from build123d import *
from build123d.topology import SkipClean

# Parameters (mm, degrees)
SKETCH1_W                = 60
SKETCH1_H                = 30
SKETCH1_R                = 11.5
BOSS_EXTRUDE1_DEPTH      = 5
SKETCH2_R                = 1.6
CUT_EXTRUDE1_DEPTH       = 68.268120235
FILLET1_R                = 5
SKETCH6_R                = 1.6
SKETCH6_R_2              = 11.5
BOSS_EXTRUDE4_DEPTH      = 3
FILLET1_OF_MIRROR1_R     = 5
SKETCH7_W                = 8
SKETCH7_H                = 5
BOSS_EXTRUDE5_DEPTH      = 8
CHAMFER1_SIZE            = 7
CHAMFER1_OF_MIRROR2_SIZE = 7


with BuildPart() as part:
    # Sketch1 → Boss-Extrude1 (new body)
    with BuildSketch(Plane(origin=(0, 0, 0), x_dir=(1, 0, 0), z_dir=(0, 1, 0))):
        with Locations((30, 15)):
            Rectangle(SKETCH1_W, SKETCH1_H)
        with Locations(Location((22, 15, 0), (0, 0, 270))):
            Circle(SKETCH1_R, mode=Mode.SUBTRACT)
    boss_extrude1 = extrude(amount=BOSS_EXTRUDE1_DEPTH)

    # Sketch2 → Cut-Extrude1 (cut, through all)
    with BuildSketch(Plane(origin=(0, 5, 0), x_dir=(1, 0, 0), z_dir=(0, 1, 0))):
        with Locations(Location((56, 25, 0), (0, 0, 270))):
            Circle(SKETCH2_R)
        with Locations(Location((56, 5, 0), (0, 0, 270))):
            Circle(SKETCH2_R)
    cut_extrude1 = extrude(amount=-CUT_EXTRUDE1_DEPTH, mode=Mode.SUBTRACT)

    # Fillet1
    fillet1_edges = [part.edges().sort_by_distance(p)[0] for p in [
        (0, 2.5, -30),
        (0, 2.5, 0),
    ]]
    fillet(fillet1_edges, radius=FILLET1_R)

    # Sketch6 → Boss-Extrude4 (add)
    with SkipClean():  # the faces are left unmerged after this step: merging them gives an invalid solid
        with BuildSketch(Plane.XZ):
            with BuildLine():
                Line((60, -30), (60, 0))
                Line((60, 0), (5, 0))
                ThreePointArc((5, 0), (1.464466094, -1.464466094), (0, -5))
                Line((0, -5), (0, -25))
                ThreePointArc((0, -25), (1.464466094, -28.535533906), (5, -30))
                Line((5, -30), (60, -30))
            make_face()
            with Locations((56, -25)):
                Circle(SKETCH6_R, mode=Mode.SUBTRACT)
            with Locations((22, -15)):
                Circle(SKETCH6_R_2, mode=Mode.SUBTRACT)
            with Locations((56, -5)):
                Circle(SKETCH6_R, mode=Mode.SUBTRACT)
        boss_extrude4 = extrude(amount=BOSS_EXTRUDE4_DEPTH)

    # Mirror1: Boss-Extrude1, Cut-Extrude1, Boss-Extrude4 across plane
    with SkipClean():  # the faces are left unmerged after this step: merging them gives an invalid solid
        add(boss_extrude1.mirror(Plane(origin=(56, 0, 0), x_dir=(0, 0, 1), z_dir=(1, 0, 0))))
        add(cut_extrude1.mirror(Plane(origin=(56, 0, 0), x_dir=(0, 0, 1), z_dir=(1, 0, 0))), mode=Mode.SUBTRACT)
        add(boss_extrude4.mirror(Plane(origin=(56, 0, 0), x_dir=(0, 0, 1), z_dir=(1, 0, 0))))

    # Fillet1 of Mirror1
    fillet1_of_mirror1_edges = [part.edges().sort_by_distance(p)[0] for p in [
        (112, 2.5, -30),
        (112, 2.5, 0),
    ]]
    fillet(fillet1_of_mirror1_edges, radius=FILLET1_OF_MIRROR1_R)

    # Sketch7 → Boss-Extrude5 (add)
    with SkipClean():  # the faces are left unmerged after this step: merging them gives an invalid solid
        with BuildSketch(Plane(origin=(0, 5, 0), x_dir=(1, 0, 0), z_dir=(0, 1, 0))):
            with Locations((47.75, 20)):
                Rectangle(SKETCH7_W, SKETCH7_H)
            with Locations((64.25, 20)):
                Rectangle(SKETCH7_W, SKETCH7_H)
        boss_extrude5 = extrude(amount=BOSS_EXTRUDE5_DEPTH)

    # Chamfer1
    chamfer1_edges = [part.edges().sort_by_distance(p)[0] for p in [
        (43.75, 13, -20),
        (68.25, 13, -20),
    ]]
    chamfer(chamfer1_edges, length=CHAMFER1_SIZE)

    # Mirror2: Boss-Extrude5 across plane
    with SkipClean():  # the faces are left unmerged after this step: merging them gives an invalid solid
        add(boss_extrude5.mirror(Plane(origin=(0, 0, -15), x_dir=(1, 0, 0), z_dir=(0, 0, -1))))

    # Chamfer1 of Mirror2
    chamfer1_of_mirror2_edges = [part.edges().sort_by_distance(p)[0] for p in [
        (43.75, 13, -10),
        (68.25, 13, -10),
    ]]
    chamfer(chamfer1_of_mirror2_edges, length=CHAMFER1_OF_MIRROR2_SIZE)


solid = part.part
The model under review builds one solid part; all positions refer to its coordinate system, in mm. A direction names the side the tool comes from. Give positions to 0.01 mm unless a question says otherwise; leave off trailing zeros. Loops run counter-clockwise (first coordinate to the right, second up) from the corner with the lowest first, then second, coordinate; pieces in that order, holes last. Notation, with made-up numbers: (19.25, 35) -> (67.25, 35) arc R30 cw to (67.25, 66) -> close; hole circle Ø1 at (2, 21.25). An arc over 180 degrees is marked (long way). Write each question's results on one line, items separated by ' | '.
1) Draft analysis for pull direction Z (two halves, no side actions). For faces 6 (the face through (49, 8, -12.5)), 7 (the face through (110, -1, -1)), 8 (the face through (64.7, 9.55, -10.04)), state which applies: pulls with the +Z half, pulls with the -Z half, needs draft (parallel to the pull), parting line crosses it, or undercut.
Conclusion:
face 6: undercut | face 7: pulls with the +Z half | face 8: needs draft
2) Tool access review of faces 1 (the face through (49, 8, -7.5)), 2 (the face through (63, 8, -22.5)), 3 (the face through (112, 1, -15)), 4 (the face through (63, 8, -12.5)), 5 (the face through (60.25, 9, -20)): name each direction out of +Z, -Z, +X, -X, +Y, -Y from which nothing blocks a thin tool from reaching the whole face with its end or side.
Conclusion:
face 1: +Z, +X, -X, +Y | face 2: -Z, +X, -X, +Y | face 3: +Z, -Z, +X, +Y, -Y | face 4: +X, -X, +Y | face 5: +Z, -Z, +Y
3) Take a section at D-D, the plane x = 37. Give the boundary of the cut face in (y, z), plus the area to 3 significant figures.
Conclusion:
outline: (-3, -30) -> (5, -30) -> (5, 0) -> (-3, 0) -> close | area: 240 mm^2
4) For line 1 along Z through (x, y) = (56, 3.25); line 2 along X through (y, z) = (2.75, -15); line 3 along X through (y, z) = (-0.25, -11.75), list the stretches that pass through material, from the lowest coordinate up. Write a range as from..to.
Conclusion:
line 1: z = -30..-26.6, -23.4..-6.6, -3.4..0 | line 2: x = 0..10.5, 33.5..78.5, 101.5..112 | line 3: x = 0..10.97, 33.03..78.97, 101.03..112
5) Take a section at C-C, the plane x = 62.5. Give the boundary of the cut face in (y, z), plus the area to 4 significant figures.
Conclusion:
outline: (-3, -30) -> (5, -30) -> (5, -22.5) -> (11.75, -22.5) -> (11.75, -17.5) -> (5, -17.5) -> (5, -12.5) -> (11.75, -12.5) -> (11.75, -7.5) -> (5, -7.5) -> (5, 0) -> (-3, 0) -> close | area: 307.5 mm^2
6) Take a section at A-A, the plane x = 22. Give the boundary of the cut face in (y, z).
Conclusion:
outline: (-3, -30) -> (5, -30) -> (5, -26.5) -> (-3, -26.5) -> close; (-3, -3.5) -> (5, -3.5) -> (5, 0) -> (-3, 0) -> close
7) Insertion check: pin 1 Ø4 at (x, y) = (49.5, 9) entering from +Z; pin 2 Ø0.5 at (y, z) = (5.5, -20.5) entering from +X; pin 3 Ø2.5 at (y, z) = (9.5, -20) entering from +X. Each pin has a flat end and moves straight along its axis. Give the tip position at first contact, or say it passes through.
Conclusion:
pin 1: stops at z = -7.5 | pin 2: stops at x = 68.25 | pin 3: stops at x = 66
8) Take a section at B-B, the plane y = 10. Give the boundary of the cut face in (x, z), plus the area to 3 significant figures.
Conclusion:
outline: (47.75, -22.5) -> (51.75, -22.5) -> (51.75, -17.5) -> (47.75, -17.5) -> close; (47.75, -12.5) -> (51.75, -12.5) -> (51.75, -7.5) -> (47.75, -7.5) -> close; (60.25, -22.5) -> (64.25, -22.5) -> (64.25, -17.5) -> (60.25, -17.5) -> close; (60.25, -12.5) -> (64.25, -12.5) -> (64.25, -7.5) -> (60.25, -7.5) -> close | area: 80.0 mm^2
